```python
from build123d import *

# Parameters (mm, degrees)
SKETCH1_R           = 1.6
BOSS_EXTRUDE1_DEPTH = 8
CHAMFER1_SIZE       = 1


with BuildPart() as part:
    # Sketch1 → Boss-Extrude1 (new body)
    with BuildSketch(Plane.XY):
        with BuildLine():
            Line((-0.5, 3), (15.5, 3))
            ThreePointArc((15.5, 3), (17.267766953, 2.267766953), (18, 0.5))
            Line((18, 0.5), (18, -0.5))
            ThreePointArc((18, -0.5), (17.267766953, -2.267766953), (15.5, -3))
            Line((15.5, -3), (-0.5, -3))
            ThreePointArc((-0.5, -3), (-2.267766953, -2.267766953), (-3, -0.5))
            Line((-3, -0.5), (-3, 0.5))
            ThreePointArc((-3, 0.5), (-2.267766953, 2.267766953), (-0.5, 3))
        make_face()
        Circle(SKETCH1_R, mode=Mode.SUBTRACT)
        with Locations((7.5, 0)):
            Circle(SKETCH1_R, mode=Mode.SUBTRACT)
        with Locations((15, 0)):
            Circle(SKETCH1_R, mode=Mode.SUBTRACT)
    extrude(amount=BOSS_EXTRUDE1_DEPTH)

    # Chamfer1
    chamfer1_edges = [part.edges().sort_by_distance(p)[0] for p in [
        (-1.6, 0, 0),
        (-1.6, 0, 8),
        (5.9, 0, 0),
        (5.9, 0, 8),
        (13.4, 0, 0),
        (13.4, 0, 8),
    ]]
    chamfer(chamfer1_edges, length=CHAMFER1_SIZE)


solid = part.part
```
Verification items for the finished model (mm, model axes). Round coordinates to 2 decimals unless told otherwise and drop trailing zeros. Write each loop counter-clockwise with the first axis right and the second up, starting at its lowest first coordinate (ties: lowest second). Pieces come first, ordered by that corner, then holes. Notation, with made-up numbers: (19.5, -40) -> (42.5, -40) arc R13 ccw to (42.5, -33) -> close; hole circle Ø4 at (58, 0.5). An arc over 180 degrees is marked (long way). Write each question's results on one line, items separated by ' | '.
Q1. Draft check along X on faces 1 (the face through (10, -1.3, 8)), 2 (the face through (17.248, 2.287, 3.944)), 3 (the face through (-1.27, -0.97, 3.96)). Enter one of: released by +X, released by -X, zero draft, split by the parting line, or undercut.
Derived:
face 1: zero draft | face 2: released by +X | face 3: undercut
Q2. Sectioned sample at C-C, the plane z = 6.5. Record the boundary of the cut face in (x, y), and give its area (3 significant figures).
Derived:
outline: (-3, -0.5) arc R2.5 ccw to (-0.5, -3) -> (15.5, -3) arc R2.5 ccw to (18, -0.5) -> (18, 0.5) arc R2.5 ccw to (15.5, 3) -> (-0.5, 3) arc R2.5 ccw to (-3, 0.5) -> close; hole circle Ø3.2 at (0, 0); hole circle Ø3.2 at (7.5, 0); hole circle Ø3.2 at (15, 0) | area: 96.5 mm²
Q3. Sectioned sample at B-B, the plane x = 15. Record the boundary of the cut face in (y, z).
Derived:
outline: (-3, 0) -> (-2.6, 0) -> (-1.6, 1) -> (-1.6, 7) -> (-2.6, 8) -> (-3, 8) -> close; (1.6, 1) -> (2.6, 0) -> (3, 0) -> (3, 8) -> (2.6, 8) -> (1.6, 7) -> close
Q4. Sectioned sample at D-D, the plane y = -0.95. Give the number of separate pieces and of enclosed holes in the cut face, and give its area (3 significant figures).
Derived:
separate pieces: 4 | enclosed holes: 0 | area: 98.6 mm²
Q5. Thickness scan on probe 1 along X at (y, z) = (-1.2, 2); probe 2 along X at (y, z) = (-0.6, 4.5); probe 3 along Y at (x, z) = (15, 4.4). Record the ranges inside material, lowest first.
Derived:
probe 1: x = -2.9 to -1.06, 1.06 to 6.44, 8.56 to 13.94, 16.06 to 17.9 | probe 2: x = -3 to -1.48, 1.48 to 6.02, 8.98 to 13.52, 16.48 to 18 | probe 3: y = -3 to -1.6, 1.6 to 3
Q6. Go/stop test with flat-tipped pins: pin 1 Ø2.5 at (x, y) = (7.5, 0) entering from +Z; pin 2 Ø1 at (y, z) = (-2, 3) entering from -X. Record where each tip stops, or that it passes through.
Derived:
pin 1: passes through | pin 2: stops at x = -2.79
Q7. Sectioned sample at A-A, the plane y = 0. Record the boundary of the cut face in (x, z).
Derived:
outline: (-3, 0) -> (-2.6, 0) -> (-1.6, 1) -> (-1.6, 7) -> (-2.6, 8) -> (-3, 8) -> close; (1.6, 1) -> (2.6, 0) -> (4.9, 0) -> (5.9, 1) -> (5.9, 7) -> (4.9, 8) -> (2.6, 8) -> (1.6, 7) -> close; (9.1, 1) -> (10.1, 0) -> (12.4, 0) -> (13.4, 1) -> (13.4, 7) -> (12.4, 8) -> (10.1, 8) -> (9.1, 7) -> close; (16.6, 1) -> (17.6, 0) -> (18, 0) -> (18, 8) -> (17.6, 8) -> (16.6, 7) -> close
